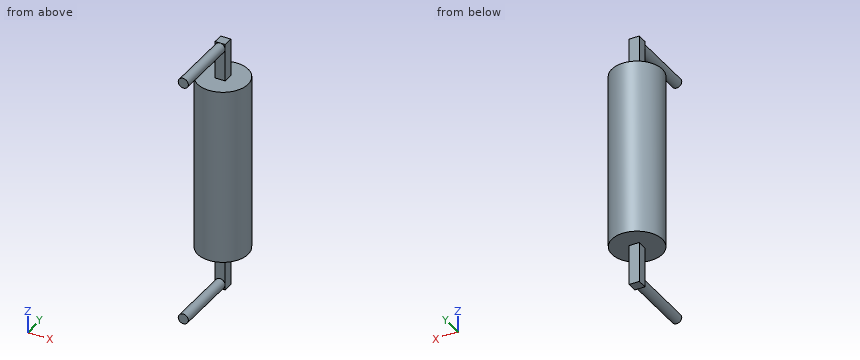
from build123d import *

# Parameters (mm, degrees)
SKETCH_1_R           = 2.5
EXTRUDE_1_DEPTH      = 17.5
EXTRUDE_2_DEPTH      = 3.75
EXTRUDE_2_DEPTH_BACK = 21.5
SKETCH_2_W           = 1
SKETCH_2_H           = 1
SKETCH_3_R           = 0.5
EXTRUDE_3_DEPTH      = 6.5


with BuildPart() as part:
    # Эскиз1 → Вытянуть1 (new body)
    with BuildSketch(Plane.XY):
        Circle(SKETCH_1_R)
    extrude(amount=EXTRUDE_1_DEPTH)

    # Эскиз2 → Вытянуть2 (add, two sides: drawn at the far end of the back side and taken through both)
    with BuildSketch(Plane.XY.offset(17.5).offset(-EXTRUDE_2_DEPTH_BACK)):
        Rectangle(SKETCH_2_W, SKETCH_2_H)
    extrude(amount=EXTRUDE_2_DEPTH + EXTRUDE_2_DEPTH_BACK)

    # Эскиз3 → Вытянуть3 (add)
    with BuildSketch(Plane.XZ.offset(0.5)):
        with Locations((0, 20.75)):
            Circle(SKETCH_3_R)
        with Locations((0, -3.5)):
            Circle(SKETCH_3_R)
    extrude(amount=EXTRUDE_3_DEPTH)


solid = part.part
The listing builds one solid part. Answer for the finished solid, in the listing's coordinates (mm). Round coordinates to 2 decimals unless told otherwise and drop trailing zeros. Order: outer loops, then holes, each group sorted by start corner. A loop starts at its lowest first (then second) coordinate and runs counter-clockwise, first axis right, second up. Notation, with made-up numbers: (23, 86.25) -> (33, 86.25) arc R21 cw to (33, 100.25) -> close; hole circle Ø11 at (36.25, -28). An arc over 180 degrees is marked (long way). One line per item, written item: value.
Item 1: Straight lines are drawn through the part: L1, parallel to Z at x = -0.05, y = -6.25; L2, parallel to Z at x = 2, y = 0.5; L3, parallel to X at y = 0.25, z = 0.25. For each, find the intervals that lie inside material, in ascending order.
Taken from the geometry:
L1: z = -4 to -3, 20.25 to 21.25
L2: z = 0 to 17.5
L3: x = -2.49 to 2.49
Item 2: Find section C-C, the plane z = 3.5. Give the vertices of the cut face in (x, y).
Taken from the geometry:
outline: circle Ø5 at (0, 0)
Item 3: Given P1, Ø0.8, axis at x = 0, z = 18.5, coming from the +Y side; P2, Ø3, axis at x = 0, z = 1, coming from the -Y side; P3, Ø0.5, axis at x = 0, z = -1.5, coming from the -Y side, each flat-ended and moving along its own axis, determine where each tip first touches the part or whether it passes through.
Taken from the geometry:
P1: stops at y = 0.5
P2: stops at y = -2.5
P3: stops at y = -0.5
Item 4: Find section B-B, the plane y = 0. Give the vertices of the cut face in (x, z), then the cut area to 4 significant figures.
Taken from the geometry:
outline: (-2.5, 0) -> (-0.5, 0) -> (-0.5, -4) -> (0.5, -4) -> (0.5, 0) -> (2.5, 0) -> (2.5, 17.5) -> (0.5, 17.5) -> (0.5, 21.25) -> (-0.5, 21.25) -> (-0.5, 17.5) -> (-2.5, 17.5) -> close
area: 95.25 mm2
Item 5: Find section D-D, the plane y = -2.75. Give the vertices of the cut face in (x, z).
Taken from the geometry:
outline: circle Ø1 at (0, -3.5); circle Ø1 at (0, 20.75)
Item 6: Find section A-A, the plane y = -1.75. Give the vertices of the cut face in (x, z).
Taken from the geometry:
outline: (-1.79, 0) -> (1.79, 0) -> (1.79, 17.5) -> (-1.79, 17.5) -> close; circle Ø1 at (0, -3.5); circle Ø1 at (0, 20.75)
